The drawing under review shows one solid part. Ordinate dimensions are in mm from its lowest x, y, z. A direction names the side the tool comes from. Round coordinates to 2 decimals unless told otherwise and drop trailing zeros. Order: outer loops, then holes, each group sorted by start corner. A loop starts at its lowest first (then second) coordinate and runs counter-clockwise, first axis right, second up. Notation, with made-up numbers: M 87,55.5 L 113,55.5 A9 cw 113,61.5 Z; hole C -35,34.25 d6. An arc over 180 degrees is marked long. Use a Markdown table: item, result.
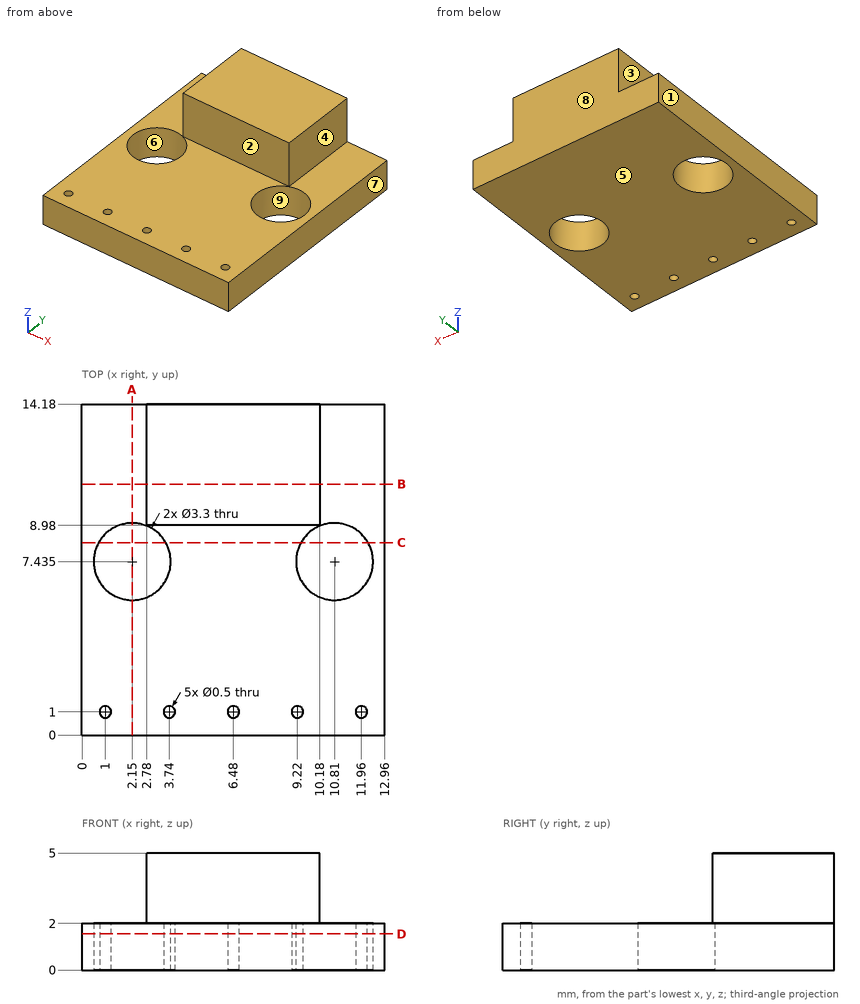
Q1. Clearance check with flat-ended pins moving along their axes: pin 1 (2 mm diameter, centred on x = 2.15, y = 7.435, fed in from +Z); pin 2 (1 mm diameter, centred on x = 7.5, y = 4.5, fed in from +Z); pin 3 (0.9 mm diameter, centred on x = 7.5, z = 3, fed in from -Y); pin 4 (1.5 mm diameter, centred on y = 11.5, z = 4, fed in from +X). State where each tip first meets the part, or that it passes through.
Determined:
| item | result |
|---|---|
| pin 1 | passes through |
| pin 2 | stops at z = 2 |
| pin 3 | stops at y = 8.98 |
| pin 4 | stops at x = 10.18 |
Q2. Wall thickness on line 1 along Y through (x, z) = (6.48, 0.55); line 2 along X through (y, z) = (8.5, 1.3); line 3 along Y through (x, z) = (11.96, 1.2): over which ranges is each line inside the solid? List them lowest first. Write a range as [from, to].
Determined:
| item | result |
|---|---|
| line 1 | y = [0, 0.75], [1.25, 14.18] |
| line 2 | x = [0, 0.89], [3.41, 9.55], [12.07, 12.96] |
| line 3 | y = [0, 0.75], [1.25, 6.25], [8.62, 14.18] |
Q3. Add section D-D (z = 1.55). Write out the cut boundary in (x, y) (3 decimals), then the cut area to 3 significant figures.
Determined:
| item | result |
|---|---|
| outline | M 0,0 L 12.96,0 L 12.96,14.18 L 0,14.18 Z; hole C 2.15,7.435 d3.3; hole C 1,1 d0.5; hole C 3.74,1 d0.5; hole C 6.48,1 d0.5; hole C 9.22,1 d0.5; hole C 10.81,7.435 d3.3; hole C 11.96,1 d0.5 |
| area | 166 mm^2 |
Q4. Add section C-C (y = 8.25). Write out the cut boundary in (x, z).
Determined:
| item | result |
|---|---|
| outline | M 0,0 L 0.72,0 L 0.72,2 L 0,2 Z; M 3.58,0 L 9.38,0 L 9.38,2 L 3.58,2 Z; M 12.24,0 L 12.96,0 L 12.96,2 L 12.24,2 Z |
Q5. Add section B-B (y = 10.75). Write out the cut boundary in (x, z).
Determined:
| item | result |
|---|---|
| outline | M 0,0 L 12.96,0 L 12.96,2 L 10.18,2 L 10.18,5 L 2.78,5 L 2.78,2 L 0,2 Z |
Q6. Machinability: for the marked faces 1, 2, 3, 4 and 5, which of the approach directions +Z, -Z, +X, -X, +Y, -Y give a long, thin tool a straight path to every point of the face, cutting with its end or side? Answer none if there is none.
Determined:
| item | result |
|---|---|
| face 1 | +Z, -Z, -X, +Y, -Y |
| face 2 | +Z, +X, -X, -Y |
| face 3 | +Z, -X, +Y, -Y |
| face 4 | +Z, +X, +Y, -Y |
| face 5 | -Z, +X, -X, +Y, -Y |
Q7. Draft analysis for pull direction Y (two halves, no side actions). For the marked faces 6, 7, 8 and 9, state which applies: pulls with the +Y half, pulls with the -Y half, needs draft (parallel to the pull), parting line crosses it, or undercut.
Determined:
| item | result |
|---|---|
| face 6 | undercut |
| face 7 | needs draft |
| face 8 | pulls with the +Y half |
| face 9 | undercut |
Q8. Add section A-A (x = 2.15). Write out the cut boundary in (y, z) (3 decimals), then the cut area to 3 significant figures.
Determined:
| item | result |
|---|---|
| outline | M 0,0 L 5.785,0 L 5.785,2 L 0,2 Z; M 9.085,0 L 14.18,0 L 14.18,2 L 9.085,2 Z |
| area | 21.8 mm^2 |
